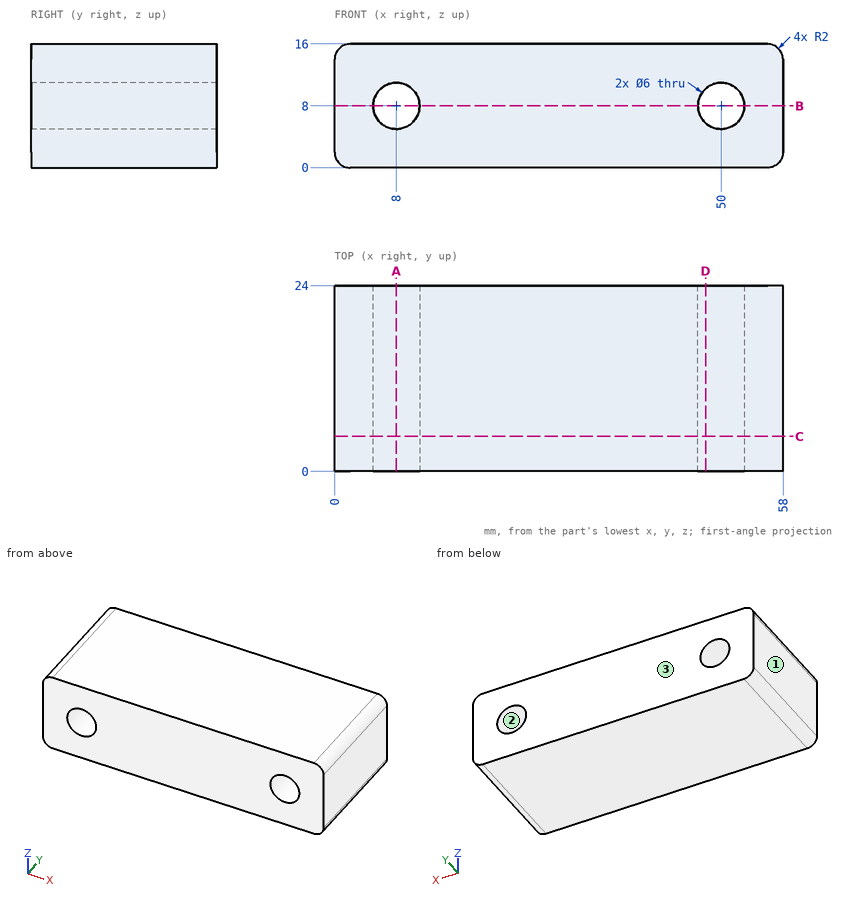
Input: dimensioned drawing with shaded views. Units: mm. Origin: part minimum x, y, z. Give positions to 0.01 mm unless a question says otherwise; leave off trailing zeros. Loops run counter-clockwise (first coordinate to the right, second up) from the corner with the lowest first, then second, coordinate; pieces in that order, holes last. Notation, with made-up numbers: (79.25, -34) -> (91.25, -34) arc R26 ccw to (91.25, -12) -> close; hole circle Ø3 at (-27, -22.75). An arc over 180 degrees is marked (long way). Return JSON: item names as keys, results as strings.
Item 1: Pin query (flat end, axial travel): P1, Ø5.5, axis at x = 50, z = 8, coming from the +Y side. Return the tip coordinate at first contact, or that it passes through.
Filled in:
{"P1": "through"}
Item 2: Line query: line 1 (X direction, y = 21.5, z = 7.75); line 2 (Z direction, x = 8, y = 13.5); line 3 (X direction, y = 7, z = 9.5). Output: solid intervals per line, ascending.
Filled in:
{"line 1": "0 to 5.01, 10.99 to 47.01, 52.99 to 58", "line 2": "0 to 5, 11 to 16", "line 3": "0 to 5.4, 10.6 to 47.4, 52.6 to 58"}
Item 3: Section A-A, the plane x = 8. Output: boundary loops of the cut face in (y, z), plus the area to 3 significant figures.
Filled in:
{"outline": "(0, 0) -> (24, 0) -> (24, 5) -> (0, 5) -> close; (0, 11) -> (24, 11) -> (24, 16) -> (0, 16) -> close", "area": "240 mm^2"}
Item 4: Section D-D, the plane x = 48. Output: boundary loops of the cut face in (y, z), plus the area to 3 significant figures.
Filled in:
{"outline": "(0, 0) -> (24, 0) -> (24, 5.76) -> (0, 5.76) -> close; (0, 10.24) -> (24, 10.24) -> (24, 16) -> (0, 16) -> close", "area": "277 mm^2"}
Item 5: Section B-B, the plane z = 8. Output: boundary loops of the cut face in (x, y), plus the area to 3 significant figures.
Filled in:
{"outline": "(0, 0) -> (5, 0) -> (5, 24) -> (0, 24) -> close; (11, 0) -> (47, 0) -> (47, 24) -> (11, 24) -> close; (53, 0) -> (58, 0) -> (58, 24) -> (53, 24) -> close", "area": "1,100 mm^2"}
Item 6: Section C-C, the plane y = 4.5. Output: boundary loops of the cut face in (x, z).
Filled in:
{"outline": "(0, 2) arc R2 ccw to (2, 0) -> (56, 0) arc R2 ccw to (58, 2) -> (58, 14) arc R2 ccw to (56, 16) -> (2, 16) arc R2 ccw to (0, 14) -> close; hole circle Ø6 at (8, 8); hole circle Ø6 at (50, 8)"}
Item 7: Mould query, pull axis X, two halves, no side actions, for the marked faces 1, 2 and 3. Classes: released by +X, released by -X, zero draft, split by the parting line, or undercut.
Filled in:
{"face 1": "released by -X", "face 2": "undercut", "face 3": "zero draft"}
